from build123d import *

# Parameters (mm, degrees)
CROQUIS1_W                 = 30
CROQUIS1_H                 = 70
SALIENTE_EXTRUIR1_DEPTH    = 200
CROQUIS5_R                 = 5
CORTAR_EXTRUIR2_DEPTH      = 20
CORTAR_EXTRUIR3_DEPTH      = 30
CORTAR_EXTRUIR3_DEPTH_BACK = 30
CROQUIS6_R                 = 40
CROQUIS7_W                 = 150
CROQUIS7_H                 = 60
CORTAR_EXTRUIR4_DEPTH      = 208.923327371
CROQUIS8_R                 = 5
CORTAR_EXTRUIR5_DEPTH      = 213.832138987


with BuildPart() as part:
    # Croquis1 → Saliente-Extruir1 (new body)
    with BuildSketch(Plane.XY):
        with Locations((4.937888199, 13.291925466)):
            Rectangle(CROQUIS1_W, CROQUIS1_H)
    extrude(amount=SALIENTE_EXTRUIR1_DEPTH)

    # Croquis5 → Cortar-Extruir2 (cut)
    with BuildSketch(Plane(origin=(0, 0, 0), x_dir=(-1, 0, 0), z_dir=(0, 0, -1))):
        with Locations((-4.937888199, 13.291925466)):
            Circle(CROQUIS5_R)
    extrude(amount=-CORTAR_EXTRUIR2_DEPTH, mode=Mode.SUBTRACT)

    # Croquis6 → Cortar-Extruir3 (cut, two sides: drawn at the far end of the back side and taken through both)
    with BuildSketch(Plane(origin=(0, 13.291925466, 0), x_dir=(-1, 0, 0), z_dir=(0, -1, 0)).offset(-CORTAR_EXTRUIR3_DEPTH_BACK)):
        with Locations((-7.25559109, -200)):
            Circle(CROQUIS6_R)
    extrude(amount=CORTAR_EXTRUIR3_DEPTH + CORTAR_EXTRUIR3_DEPTH_BACK, mode=Mode.SUBTRACT)

    # Croquis7 → Cortar-Extruir4 (cut, through all)
    with BuildSketch(Plane.ZY.offset(10.062111801)):
        with Locations((80, 13.291925466)):
            Rectangle(CROQUIS7_W, CROQUIS7_H)
    extrude(amount=-CORTAR_EXTRUIR4_DEPTH, mode=Mode.SUBTRACT)

    # Croquis8 → Cortar-Extruir5 (cut, through all)
    with BuildSketch(Plane(origin=(0, -21.708074534, 0), x_dir=(-1, 0, 0), z_dir=(0, -1, 0))):
        with Locations(Location((-4.937888199, -180, 0), (0, 0, 90))):
            Circle(CROQUIS8_R)
    extrude(amount=-CORTAR_EXTRUIR5_DEPTH, mode=Mode.SUBTRACT)


solid = part.part
Geometry check sheet. Reference: the model listing, model coordinates, mm. A direction names the side the tool comes from. Round coordinates to 2 decimals unless told otherwise and drop trailing zeros. Loops run counter-clockwise (first coordinate to the right, second up) from the corner with the lowest first, then second, coordinate; pieces in that order, holes last. Notation, with made-up numbers: (-30, 27.25) - (-23, 27.25) arc R32 cw to (-23, 54.25) - close; hole circle Ø9 at (-16.5, 59.25). An arc over 180 degrees is marked (long way). One line per question, with ' | ' between items. Start each with the question number.
1. Draft check along X on faces 4 (the face through (5, 46, 185)), 5 (the face through (19.938, -18, 92)), 6 (the face through (5, -16.708, 79)), 7 (the face through (4.539, 13.712, 160.092)). Enter one of: released by +X, released by -X, zero draft, split by the parting line, or undercut.
2. Cross-section at B-B on z = 180. Record the cut outline in (x, y), then the cut area to 3 significant figures.
3. Cross-section at C-C on y = 11. Record the cut outline in (x, z).
4. Depth check by flat-ended pin: pin 1 (1 mm diameter, centred on x = 12, y = -13.5, fed in from +Z); pin 2 (16 mm diameter, centred on x = 4.94, y = 13.29, fed in from +Z); pin 3 (4 mm diameter, centred on x = 15.5, y = 39.5, fed in from +Z). Enter the tip coordinate at first touch or a pass-through.
5. Scan lines: line 1 (Y direction, x = 1, z = 124.5); line 2 (X direction, y = -19, z = 180); line 3 (Z direction, x = 7, y = 9). Record each from-to range of solid material in increasing order. Write a range as [from, to].
6. Cross-section at D-D on x = 14. Record the cut outline in (y, z), then the cut area to 3 significant figures.
7. Tool access check on faces 1 (the face through (5, 6, 5)), 2 (the face through (-10.062, -18, 92)), 3 (the face through (6.02, 8.41, 2.46)). Record the directions out of +Z, -Z, +X, -X, +Y, -Y that give a thin tool (end or side, any length) a straight path to the whole face; none if there is none.
8. Cross-section at A-A on z = 37. Record the cut outline in (x, y), then the cut area to 3 significant figures.
Taken from the geometry:
1) face 4: undercut | face 5: released by +X | face 6: zero draft | face 7: undercut
2) outline: (-10.06, -21.71) - (-0.06, -21.71) - (-0.06, -16.71) - (-10.06, -16.71) - close; (-10.06, 43.29) - (-0.06, 43.29) - (-0.06, 48.29) - (-10.06, 48.29) - close; (9.94, -21.71) - (19.94, -21.71) - (19.94, -16.71) - (9.94, -16.71) - close; (9.94, 43.29) - (19.94, 43.29) - (19.94, 48.29) - (9.94, 48.29) - close | area: 200 mm²
3) outline: (-10.06, 0) - (0.49, 0) - (0.49, 5) - (-10.06, 5) - close; (-10.06, 155) - (19.94, 155) - (19.94, 162.06) arc R40 cw to (-10.06, 163.94) - close; (9.38, 0) - (19.94, 0) - (19.94, 5) - (9.38, 5) - close
4) pin 1: z = 160.35 | pin 2: z = 161.35 | pin 3: z = 161.33
5) line 1: [-21.71, -16.71], [43.29, 48.29] | line 2: [-10.06, -0.06], [9.94, 19.94] | line 3: [155, 160]
6) outline: (-21.71, 0) - (48.29, 0) - (48.29, 200) - (43.29, 200) - (43.29, 160.57) - (-16.71, 160.57) - (-16.71, 200) - (-21.71, 200) - close; hole (-16.71, 5) - (43.29, 5) - (43.29, 155) - (-16.71, 155) - close | area: 2,630 mm²
7) face 1: +X, -X | face 2: +Z, -Z, -X, +Y, -Y | face 3: -Z
8) outline: (-10.06, -21.71) - (19.94, -21.71) - (19.94, -16.71) - (-10.06, -16.71) - close; (-10.06, 43.29) - (19.94, 43.29) - (19.94, 48.29) - (-10.06, 48.29) - close | area: 300 mm²
